from build123d import *

# Parameters (mm, degrees)
SKETCH1_R                      = 6.2
BOSS_EXTRUDE1_DEPTH            = 13.5
F_2_7_2_7_DIAMETER_HOLE1_D     = 2.7
F_2_7_2_7_DIAMETER_HOLE1_DEPTH = 4
F_2_7_2_7_DIAMETER_HOLE1_TIP   = 0.811161836


with BuildPart() as part:
    # Sketch1 → Boss-Extrude1 (new body)
    with BuildSketch(Plane.XY):
        with BuildLine():
            Line((-9.5, 8.25), (-9.5, -8.25))
            Line((-9.5, -8.25), (0, -8.25))
            ThreePointArc((0, -8.25), (8.25, 0), (0, 8.25))
            Line((0, 8.25), (-9.5, 8.25))
        make_face()
        Circle(SKETCH1_R, mode=Mode.SUBTRACT)
    extrude(amount=BOSS_EXTRUDE1_DEPTH)

    # Ø2.7 (2.7) Diameter Hole1
    with Locations(Plane.ZY.offset(9.5)):
        with Locations((2.5, -5), (2.5, 5), (11, 5), (11, -5)):
            Hole(F_2_7_2_7_DIAMETER_HOLE1_D / 2, depth=F_2_7_2_7_DIAMETER_HOLE1_DEPTH)
            with Locations((0, 0, -(F_2_7_2_7_DIAMETER_HOLE1_DEPTH + F_2_7_2_7_DIAMETER_HOLE1_TIP / 2))):  # 118° drill point
                Cone(0, F_2_7_2_7_DIAMETER_HOLE1_D / 2, F_2_7_2_7_DIAMETER_HOLE1_TIP, mode=Mode.SUBTRACT)


solid = part.part
Read the model definition and answer for the solid it produces. Units are mm, in the model's axes. A direction names the side the tool comes from. Give positions to 0.01 mm unless a question says otherwise; leave off trailing zeros. Write each loop counter-clockwise with the first axis right and the second up, starting at its lowest first coordinate (ties: lowest second). Pieces come first, ordered by that corner, then holes. Notation, with made-up numbers: (74.25, 54) - (101.25, 54) arc R15 cw to (101.25, 77) - close; hole circle Ø11 at (-38, 18.5). An arc over 180 degrees is marked (long way). Answer in a Markdown table with one row per item. Add a question column.
Item 1: Determine the mould class of faces 1 (the face through (8.25, -0.18, 6.66)), 2 (the face through (-5, -8.25, 7)), 3 (the face through (-4.83, -4.93, 11.224)) for opening direction Y: pulls with the +Y half, pulls with the -Y half, needs draft (parallel to the pull), parting line crosses it, or undercut.
Item 2: A tool of negligible diameter and unlimited length cuts with its end or side. For faces 4 (the face through (-9.5, 0, 7)), 5 (the face through (-7.472, -5.517, 9.753)), from which of +Z, -Z, +X, -X, +Y, -Y can it reach the whole face along a straight path? Write none if from no direction.
Item 3: Section A-A, the plane x = -5.25 is taken. Write down the section's boundary in (y, z).
Item 4: Flat-ended cylindrical pins translate along their axes: P1, Ø2, axis at x = -4.5, y = 1, coming from the -Z side; P2, Ø1.5, axis at y = 4.5, z = 11.5, coming from the +X side; P3, Ø1.6, axis at y = 5, z = 2.5, coming from the -X side; P4, Ø1.6, axis at y = -5, z = 11, coming from the +X side. Find the tip coordinate at first contact, or state that the pin passes through.
Item 5: Section B-B, the plane y = 0 is taken. Write down the section's boundary in (x, z).
Item 6: Section C-C, the plane z = 4.25 is taken. Write down the section's boundary in (x, y), and give its area (3 significant figures).
Item 7: Find the intervals of material crossed by L1, parallel to Z at x = -8.35, y = 5; L2, parallel to Y at x = -8, z = 2.5; L3, parallel to X at y = 0.25, z = 5, in increasing order.
Recorded:
| question | item | result |
|---|---|---|
| 1 | face 1 | parting line crosses it |
| 1 | face 2 | pulls with the -Y half |
| 1 | face 3 | undercut |
| 2 | face 4 | +Z, -Z, -X, +Y, -Y |
| 2 | face 5 | -X |
| 3 | outline | (-8.25, 0) - (-3.3, 0) - (-3.3, 13.5) - (-8.25, 13.5) - close; (3.3, 0) - (8.25, 0) - (8.25, 13.5) - (3.3, 13.5) - close; hole circle Ø1.87 at (-5, 2.5); hole circle Ø1.87 at (-5, 11); hole circle Ø1.87 at (5, 2.5); hole circle Ø1.87 at (5, 11) |
| 4 | P1 | passes through |
| 4 | P2 | stops at x = 7.35 |
| 4 | P3 | stops at x = -5.17 |
| 4 | P4 | stops at x = 7.1 |
| 5 | outline | (-9.5, 0) - (-6.2, 0) - (-6.2, 13.5) - (-9.5, 13.5) - close; (6.2, 0) - (8.25, 0) - (8.25, 13.5) - (6.2, 13.5) - close |
| 6 | outline | (-9.5, -8.25) - (0, -8.25) arc R8.25 ccw to (0, 8.25) - (-9.5, 8.25) - close; hole circle Ø12.4 at (0, 0) |
| 6 | area | 143 mm2 |
| 7 | L1 | z = 0 to 1.15, 3.85 to 9.65, 12.35 to 13.5 |
| 7 | L2 | y = -8.25 to -6.35, -3.65 to 3.65, 6.35 to 8.25 |
| 7 | L3 | x = -9.5 to -6.19, 6.19 to 8.25 |
